Source: CAD feature listing. Evaluate the final solid. Frame: model axes, mm. A direction names the side the tool comes from. Round coordinates to 2 decimals unless told otherwise and drop trailing zeros. Order: outer loops, then holes, each group sorted by start corner. A loop starts at its lowest first (then second) coordinate and runs counter-clockwise, first axis right, second up. Notation, with made-up numbers: (19.5, -19.5) - (54.5, -19.5) arc R20 cw to (54.5, -10.5) - close; hole circle Ø8 at (-29.75, 72). An arc over 180 degrees is marked (long way). Return JSON: item names as keys, results as strings. Group by question number.
1) Access query for faces 1 (the flat face through (20, 2, -30)), 2 (the cylindrical face through (-49.14, 1.97, 29.1)). Directions: +Z, -Z, +X, -X, +Y, -Y. A direction counts if a zero-diameter tool reaches every point of the face in a straight line with its end or side. Return the directions, or none.
2) Section A-A, the plane z = -40. Return loops of the section in (x, y).
3) Mould query, pull axis X, two halves, no side actions, for faces 3 (the flat face through (-50, 2, 13)), 4 (the cylindrical face through (-29.26, 1.97, 10.37)), 5 (the cylindrical face through (9.04, 1.97, -37.69)), 6 (the cylindrical face through (27.11, 1.97, -38.66)). Classes: pulls with the +X half, pulls with the -X half, needs draft (parallel to the pull), parting line crosses it, or undercut.
4) Contact query for a flat-ended pin moving along its axis: P1, Ø1.2, axis at x = 22, y = 3, coming from the +Z side. Output: stop coordinate, or through.
5) Section C-C, the plane z = 25. Return loops of the section in (x, y), plus the area to 3 significant figures.
6) Section B-B, the plane x = 25. Return loops of the section in (y, z), plus the area to 3 significant figures.
7) Ray query, line 1 (X direction, y = 1.1, z = -40); line 2 (X direction, y = 2.8, z = 25); line 3 (X direction, y = 3.55, z = -39.5). Return the intervals inside material, ascending. Write a range as from..to.
8) Section D-D, the plane y = 2.85. Return loops of the section in (x, z), plus the area to 3 significant figures.
```python
from build123d import *

# Parameters (mm, degrees)
SKETCH1_R           = 2.5
BOSS_EXTRUDE1_DEPTH = 4


with BuildPart() as part:
    # Sketch1 → Boss-Extrude1 (new body)
    with BuildSketch(Plane(origin=(0, 0, 0), x_dir=(1, 0, 0), z_dir=(0, 1, 0))):
        with BuildLine():
            Line((-50, 0), (-50, -27))
            ThreePointArc((-50, -27), (-49.121320344, -29.121320344), (-47, -30))
            Line((-47, -30), (-33, -30))
            ThreePointArc((-33, -30), (-30.878679656, -29.121320344), (-30, -27))
            Line((-30, -27), (-30, -14.142135624))
            ThreePointArc((-30, -14.142135624), (-29.238795325, -10.3153013), (-27.071067812, -7.071067812))
            Line((-27.071067812, -7.071067812), (7.071067812, 27.071067812))
            ThreePointArc((7.071067812, 27.071067812), (10.3153013, 29.238795325), (14.142135624, 30))
            Line((14.142135624, 30), (27, 30))
            ThreePointArc((27, 30), (29.121320344, 30.878679656), (30, 33))
            Line((30, 33), (30, 47))
            ThreePointArc((30, 47), (29.121320344, 49.121320344), (27, 50))
            Line((27, 50), (0, 50))
            ThreePointArc((0, 50), (-35.355339059, 35.355339059), (-50, 0))
        make_face()
        with Locations(Location((-40, -10, 0), (0, 0, 270))):
            Circle(SKETCH1_R, mode=Mode.SUBTRACT)
        with Locations(Location((-40, -25, 0), (0, 0, 270))):
            Circle(SKETCH1_R, mode=Mode.SUBTRACT)
        with Locations(Location((10, 40, 0), (0, 0, 270))):
            Circle(SKETCH1_R, mode=Mode.SUBTRACT)
        with Locations(Location((25, 40, 0), (0, 0, 270))):
            Circle(SKETCH1_R, mode=Mode.SUBTRACT)
    extrude(amount=BOSS_EXTRUDE1_DEPTH)


solid = part.part
```
Geometry check:
{
 "1": {"face 1": "+Z, +X, +Y, -Y", "face 2": "+Z, -X, +Y, -Y"},
 "2": {"outline": "(-30, 0) - (7.5, 0) - (7.5, 4) - (-30, 4) - close; (12.5, 0) - (22.5, 0) - (22.5, 4) - (12.5, 4) - close; (27.5, 0) - (30, 0) - (30, 4) - (27.5, 4) - close"},
 "3": {"face 3": "pulls with the -X half", "face 4": "pulls with the +X half", "face 5": "undercut", "face 6": "undercut"},
 "4": {"P1": "z = -30"},
 "5": {"outline": "(-50, 0) - (-42.5, 0) - (-42.5, 4) - (-50, 4) - close; (-37.5, 0) - (-30, 0) - (-30, 4) - (-37.5, 4) - close", "area": "60.0 mm2"},
 "6": {"outline": "(0, -50) - (4, -50) - (4, -42.5) - (0, -42.5) - close; (0, -37.5) - (4, -37.5) - (4, -30) - (0, -30) - close", "area": "60.0 mm2"},
 "7": {"line 1": "-30..7.5, 12.5..22.5, 27.5..30", "line 2": "-50..-42.5, -37.5..-30", "line 3": "-30.66..7.55, 12.45..22.55, 27.45..30"},
 "8": {"outline": "(-50, 0) arc R50 ccw to (0, -50) - (27, -50) arc R3 ccw to (30, -47) - (30, -33) arc R3 ccw to (27, -30) - (14.14, -30) arc R10 cw to (7.07, -27.07) - (-27.07, 7.07) arc R10 cw to (-30, 14.14) - (-30, 27) arc R3 ccw to (-33, 30) - (-47, 30) arc R3 ccw to (-50, 27) - close; hole circle Ø5 at (-40, 10); hole circle Ø5 at (-40, 25); hole circle Ø5 at (10, -40); hole circle Ø5 at (25, -40)", "area": "2,980 mm2"}
}
